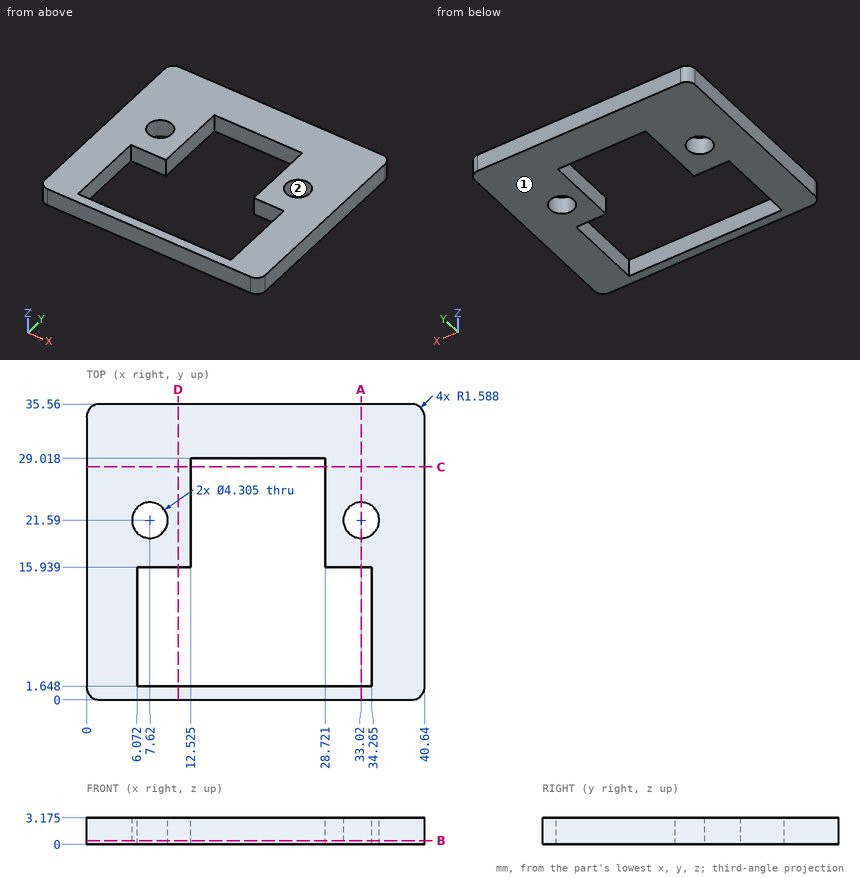
Design review of the part shown in the three views and the two pictorial views. Dimensions are in mm from the part's minimum x, y and z. Round coordinates to 2 decimals unless told otherwise and drop trailing zeros. Write each loop counter-clockwise with the first axis right and the second up, starting at its lowest first coordinate (ties: lowest second). Pieces come first, ordered by that corner, then holes.
1) Take a section at C-C on y = 28. Give the boundary of the cut face in (x, z) (1 decimal).
Answer below:
outline: (0, 0) - (12.5, 0) - (12.5, 3.2) - (0, 3.2) - close; (28.7, 0) - (40.6, 0) - (40.6, 3.2) - (28.7, 3.2) - close
2) Take a section at B-B on z = 0.45. Give the boundary of the cut face in (x, y) (1 decimal).
Answer below:
outline: (0, 1.6) arc R1.6 ccw to (1.6, 0) - (39.1, 0) arc R1.6 ccw to (40.6, 1.6) - (40.6, 34) arc R1.6 ccw to (39.1, 35.6) - (1.6, 35.6) arc R1.6 ccw to (0, 34) - close; hole circle Ø4.3 at (7.6, 21.6); hole (6.1, 1.6) - (34.3, 1.6) - (34.3, 15.9) - (28.7, 15.9) - (28.7, 29) - (12.5, 29) - (12.5, 15.9) - (6.1, 15.9) - close; hole circle Ø4.3 at (33, 21.6)
3) Mouldability with a two-part tool opening along Y and no side actions: class the marked faces 1 and 2 as +Y half, -Y half, draft (parallel to the pull), parting line (faces both ways), or undercut.
Answer below:
face 1: draft
face 2: undercut
4) Take a section at A-A on x = 33.02. Give the boundary of the cut face in (y, z) (1 decimal).
Answer below:
outline: (0, 0) - (1.6, 0) - (1.6, 3.2) - (0, 3.2) - close; (15.9, 0) - (19.4, 0) - (19.4, 3.2) - (15.9, 3.2) - close; (23.7, 0) - (35.6, 0) - (35.6, 3.2) - (23.7, 3.2) - close
5) Take a section at D-D on x = 11. Give the boundary of the cut face in (y, z) (1 decimal).
Answer below:
outline: (0, 0) - (1.6, 0) - (1.6, 3.2) - (0, 3.2) - close; (15.9, 0) - (35.6, 0) - (35.6, 3.2) - (15.9, 3.2) - close
6) Insertion check: pin 1 Ø4 at (x, y) = (33.02, 21.59) entering from +Z. The pin has a flat end and moves straight along its axis. Give the tip position at first contact, or say it passes through.
Answer below:
pin 1: passes through
7) For line 1 along Y through (x, z) = (33, 1.3); line 2 along X through (y, z) = (17.5, 1.7) (1 decimal); line 3 along X through (y, z) = (15.5, 1.55) (1 decimal), list the stretches that pass through material, from the lowest coordinate up.
Answer below:
line 1: y = 0 to 1.65, 15.94 to 19.44, 23.74 to 35.56
line 2: x = 0 to 12.5, 28.7 to 40.6
line 3: x = 0 to 6.1, 34.3 to 40.6
